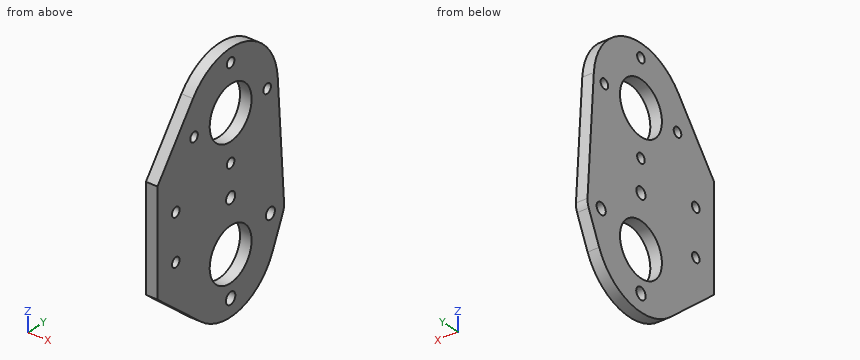
from build123d import *

# Parameters (mm, degrees)
SKETCH1_R           = 2.6289
SKETCH1_R_2         = 14.5542
SKETCH1_R_3         = 3.175
SKETCH1_R_4         = 3.2639
CORE_GEOMETRY_DEPTH = 6.35


with BuildPart() as part:
    # Sketch1 → Core geometry (new body)
    with BuildSketch(Plane(origin=(0, 0, 0), x_dir=(0, 0, -1), z_dir=(1, 0, 0))):
        with BuildLine():
            Line((76.2, 0), (101.94847561, 30.201219512))
            ThreePointArc((101.94847561, 30.201219512), (108.748010679, 57.836283003), (90.672243723, 79.818026797))
            Line((90.672243723, 79.818026797), (74.257168903, 87.106738525))
            ThreePointArc((74.257168903, 87.106738525), (72.055689407, 87.779865373), (69.757012949, 87.905158095))
            Line((69.757012949, 87.905158095), (4.07592642, 83.518510516))
            ThreePointArc((4.07592642, 83.518510516), (-25.155846577, 60.194220655), (-13.526294854, 24.651674645))
            Line((-13.526294854, 24.651674645), (19.05, 0))
            Line((19.05, 0), (76.2, 0))
        make_face()
        with Locations((38.1, 12.7)):
            Circle(SKETCH1_R, mode=Mode.SUBTRACT)
        with Locations((63.5, 12.7)):
            Circle(SKETCH1_R, mode=Mode.SUBTRACT)
        with Locations((77.7875, 50.8)):
            Circle(SKETCH1_R_2, mode=Mode.SUBTRACT)
        with Locations((6.2611, 50.8)):
            Circle(SKETCH1_R_2, mode=Mode.SUBTRACT)
        with Locations((6.2611, 76.2)):
            Circle(SKETCH1_R, mode=Mode.SUBTRACT)
        with Locations((6.2611, 25.4)):
            Circle(SKETCH1_R, mode=Mode.SUBTRACT)
        with Locations((31.6611, 50.8)):
            Circle(SKETCH1_R, mode=Mode.SUBTRACT)
        with Locations((-19.1389, 50.8)):
            Circle(SKETCH1_R, mode=Mode.SUBTRACT)
        with Locations((49.2125, 50.8)):
            Circle(SKETCH1_R_3, mode=Mode.SUBTRACT)
        with Locations((70.391745786, 78.401330486)):
            Circle(SKETCH1_R_3, mode=Mode.SUBTRACT)
        with Locations((100.0125, 50.8)):
            Circle(SKETCH1_R_4, mode=Mode.SUBTRACT)
    extrude(amount=CORE_GEOMETRY_DEPTH)


solid = part.part
Could you check a few things on this model? Use its own coordinates, in mm. Give positions to 0.01 mm unless a question says otherwise; leave off trailing zeros. Order: outer loops, then holes, each group sorted by start corner. A loop starts at its lowest first (then second) coordinate and runs counter-clockwise, first axis right, second up. Notation, with made-up numbers: (38, 84) - (43, 84) arc R18 cw to (43, 101) - close; hole circle Ø4 at (-7.5, 83). An arc over 180 degrees is marked (long way). Return JSON: item names as keys, results as strings. Group by question number.
Q1. Suppose I cut it at D-D, the plane x = 3.25. State how many separate pieces and enclosed holes the cut face has, and give its area (3 significant figures).
Q2. Will these pins go through, and if not, where does the flat tip stop? pin 1 Ø3 at (x, z) = (4.5, -46) entering from +Y; pin 2 Ø1 at (x, z) = (2.5, -20.5) entering from +Y; pin 3 Ø3 at (x, z) = (3, -6) entering from +Y.
Q3. Suppose I cut it at B-B, the plane z = -31.5. Please give me the cut outline in (x, y).
Q4. Suppose I cut it at A-A, the plane y = 50.8. Please give me the cut outline in (x, z).
Q5. Suppose I cut it at C-C, the plane y = 12.7. Please give me the cut outline in (x, z), and give its area (3 significant figures).
Q6. Please list where these lines run through material, in increasing order: line 1 along Z through (x, y) = (2.25, 63); line 2 along Z through (x, y) = (5.75, 38); line 3 along Y through (x, z) = (2, -67). Write a range as [from, to].
Resolved:
{
 "1": {"separate pieces": "1", "enclosed holes": "11", "area": "8,020 mm2"},
 "2": {"pin 1": "stops at y = 86.42", "pin 2": "stops at y = 84.65", "pin 3": "stops at y = 83.75"},
 "3": {"outline": "(0, 0) - (6.35, 0) - (6.35, 48.18) - (0, 48.18) - close; (0, 53.42) - (6.35, 53.42) - (6.35, 85.35) - (0, 85.35) - close"},
 "4": {"outline": "(0, -109.54) - (6.35, -109.54) - (6.35, -103.28) - (0, -103.28) - close; (0, -96.75) - (6.35, -96.75) - (6.35, -92.34) - (0, -92.34) - close; (0, -63.23) - (6.35, -63.23) - (6.35, -52.39) - (0, -52.39) - close; (0, -46.04) - (6.35, -46.04) - (6.35, -34.29) - (0, -34.29) - close; (0, -29.03) - (6.35, -29.03) - (6.35, -20.82) - (0, -20.82) - close; (0, 8.29) - (6.35, 8.29) - (6.35, 16.51) - (0, 16.51) - close; (0, 21.77) - (6.35, 21.77) - (6.35, 26.53) - (0, 26.53) - close"},
 "5": {"outline": "(0, -87.03) - (6.35, -87.03) - (6.35, -66.13) - (0, -66.13) - close; (0, -60.87) - (6.35, -60.87) - (6.35, -40.73) - (0, -40.73) - close; (0, -35.47) - (6.35, -35.47) - (6.35, -2.27) - (0, -2.27) - close", "area": "471 mm2"},
 "6": {"line 1": "z = [-107.1, -85.72], [-69.85, -14.2], [1.68, 24.18]", "line 2": "z = [-106.84, -84.71], [-70.86, -13.19], [0.67, 23.93]", "line 3": "y = [0, 41.03], [60.57, 87.72]"}
}
